Can you work these out from the model? Positions are in its coordinate system, mm. Face numbers are marked on the shaded views. A direction names the side the tool comes from. Round coordinates to 2 decimals unless told otherwise and drop trailing zeros. Loops run counter-clockwise (first coordinate to the right, second up) from the corner with the lowest first, then second, coordinate; pieces in that order, holes last. Notation, with made-up numbers: (47.25, 50) -> (60.25, 50) arc R24 cw to (60.25, 89) -> close; hole circle Ø11 at (-35.5, 86.25). An arc over 180 degrees is marked (long way). Use a Markdown table: item, result.
from build123d import *

# Parameters (mm, degrees)
BOSS_EXTRUDE1_DEPTH = 11
SKETCH2_R           = 3
CUT_EXTRUDE1_DEPTH  = 60
SKETCH4_R           = 2
CUT_EXTRUDE2_DEPTH  = 11


with BuildPart() as part:
    # Sketch1 → Boss-Extrude1 (new body)
    with BuildSketch(Plane.XY):
        Polygon((0, 50), (50, 50), (50, 0), (0, 0), (0, 5), (45, 5), (45, 45), (0, 45), align=None)
    extrude(amount=BOSS_EXTRUDE1_DEPTH)

    # Sketch2 → Cut-Extrude1 (cut)
    with BuildSketch(Plane(origin=(0, 50, 0), x_dir=(1, 0, 0), z_dir=(0, 1, 0))):
        with Locations(Location((6, -5.5, 0), (0, 0, 270))):
            Circle(SKETCH2_R)
    extrude(amount=-CUT_EXTRUDE1_DEPTH, mode=Mode.SUBTRACT)

    # Sketch4 → Cut-Extrude2 (cut)
    with BuildSketch(Plane.ZY.offset(-45)):
        with Locations((5.5, 40)):
            Circle(SKETCH4_R)
        with Locations((5.5, 10)):
            Circle(SKETCH4_R)
    extrude(amount=-CUT_EXTRUDE2_DEPTH, mode=Mode.SUBTRACT)


solid = part.part
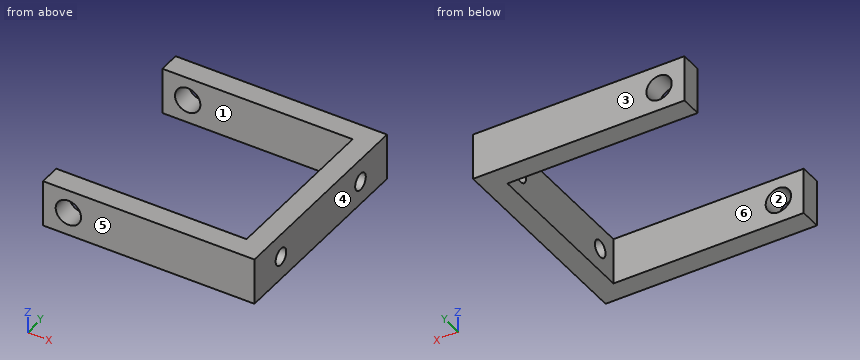
1. Will these pins go through, and if not, where does the flat tip stop? pin 1 Ø3.5 at (x, z) = (6, 5.5) entering from -Y; pin 2 Ø6.5 at (y, z) = (10, 5.5) entering from -X.
Answer sheet:
| item | result |
|---|---|
| pin 1 | passes through |
| pin 2 | stops at x = 45 |
2. I need wall thicknesses on line 1 (Y direction, x = 47.5, z = 5.5); line 2 (Y direction, x = 29.5, z = 1.5); line 3 (X direction, y = 2.45, z = 5.5). Which ranges of each line are inside material? Lowest first, please.
Answer sheet:
| item | result |
|---|---|
| line 1 | y = 0 to 8, 12 to 38, 42 to 50 |
| line 2 | y = 0 to 5, 45 to 50 |
| line 3 | x = 0 to 3, 9 to 50 |
3. I want a section at C-C (x = 15). Please give me the cut outline in (y, z), plus the area to 3 significant figures.
Answer sheet:
| item | result |
|---|---|
| outline | (0, 0) -> (5, 0) -> (5, 11) -> (0, 11) -> close; (45, 0) -> (50, 0) -> (50, 11) -> (45, 11) -> close |
| area | 110 mm² |
4. Which directions (+Z, -Z, +X, -X, +Y, -Y) give clear straight access to the entire face, cutting with the end or side of a thin tool? Please do the marked faces 1 and 2.
Answer sheet:
| item | result |
|---|---|
| face 1 | +Z, -Z, -X |
| face 2 | +Y, -Y |
5. I want a section at A-A (x = 6). Please give me the cut outline in (y, z).
Answer sheet:
| item | result |
|---|---|
| outline | (0, 0) -> (5, 0) -> (5, 2.5) -> (0, 2.5) -> close; (0, 8.5) -> (5, 8.5) -> (5, 11) -> (0, 11) -> close; (45, 0) -> (50, 0) -> (50, 2.5) -> (45, 2.5) -> close; (45, 8.5) -> (50, 8.5) -> (50, 11) -> (45, 11) -> close |
6. I want a section at B-B (z = 5.5). Please give me the cut outline in (x, y).
Answer sheet:
| item | result |
|---|---|
| outline | (0, 0) -> (3, 0) -> (3, 5) -> (0, 5) -> close; (0, 45) -> (3, 45) -> (3, 50) -> (0, 50) -> close; (9, 0) -> (50, 0) -> (50, 8) -> (45, 8) -> (45, 5) -> (9, 5) -> close; (9, 45) -> (45, 45) -> (45, 42) -> (50, 42) -> (50, 50) -> (9, 50) -> close; (45, 12) -> (50, 12) -> (50, 38) -> (45, 38) -> close |
7. If we mould it in two halves opening along Y, with no side actions, what happens to the marked faces 3, 4, 5 and 6? For each: +Y half, -Y half, draft (parallel to the pull), parting line (faces both ways), or undercut.
Answer sheet:
| item | result |
|---|---|
| face 3 | +Y half |
| face 4 | draft |
| face 5 | -Y half |
| face 6 | undercut |
8. I want a section at D-D (y = 40). Please give me the cut outline in (x, z), plus the area to 3 significant figures.
Answer sheet:
| item | result |
|---|---|
| outline | (45, 0) -> (50, 0) -> (50, 3.5) -> (45, 3.5) -> close; (45, 7.5) -> (50, 7.5) -> (50, 11) -> (45, 11) -> close |
| area | 35.0 mm² |
